Verification items for the finished model (mm, model axes). A direction names the side the tool comes from. Coordinates: 2 decimals unless noted, no trailing zeros. Write each loop counter-clockwise with the first axis right and the second up, starting at its lowest first coordinate (ties: lowest second). Pieces come first, ordered by that corner, then holes. Notation, with made-up numbers: (0.25, -19.5) -> (31.25, -19.5) arc R31 cw to (31.25, 11.5) -> close; hole circle Ø1 at (59.25, 83). An arc over 180 degrees is marked (long way). Write item = value, one per line. Start each with the question number.
(1) Section check A-A (x = 0). Record the cut outline in (y, z).
(2) Mould release check, pull along Z, two halves, no side actions. Record for faces 3 (the face through (0.29, -0.12, 76.25)), 4 (the face through (4, 0, 129.54)), 5 (the face through (0, 0, 0)): released by +Z, released by -Z, zero draft, split by the parting line, or undercut.
(3) Gauge pin test, flat ends, axial feed: pin 1 Ø2 at (x, z) = (0, 74.93) entering from -Y; pin 2 Ø8 at (x, z) = (-5.5, 101.5) entering from +Y; pin 3 Ø2 at (x, z) = (-5.5, 46.5) entering from -Y; pin 4 Ø1 at (x, y) = (5, -0.5) entering from +Z. Record the tip position at first contact, or that the pin passes through.
(4) Section check C-C (z = 125). Record the cut outline in (x, y).
(5) Section check B-B (y = 0). Record the cut outline in (x, z).
(6) Set-up check for faces 1 (the face through (0.29, -0.12, 109.27)), 2 (the face through (-2.3, -1.8, 138.3)): record each of +Z, -Z, +X, -X, +Y, -Y from which the full face is reachable in a straight line by a thin tool's end or side.
(7) Material ranges on probe 1 along Z at (x, y) = (0, 2); probe 2 along Z at (x, y) = (0, 0); probe 3 along Z at (x, y) = (0, 0.5), recorded low to high. Write a range as [from, to].
(8) Section check D-D (z = 107.95). Record the cut outline in (x, y), plus the area to 3 significant figures.
```python
from build123d import *

# Parameters (mm, degrees)
SKETCH1_R             = 8.73125
BOSS_EXTRUDE1_DEPTH   = 129.54
SKETCH2_R             = 2.921
BOSS_EXTRUDE2_DEPTH   = 17.78
F_6_32_TAPPED_HOLE1_D = 2.7051
F_6_32_TAPPED_HOLE2_D = 2.7051


with BuildPart() as part:
    # Sketch1 → Boss-Extrude1 (new body)
    with BuildSketch(Plane.XY):
        Circle(SKETCH1_R)
    extrude(amount=BOSS_EXTRUDE1_DEPTH)

    # Sketch2 → Boss-Extrude2 (add)
    with BuildSketch(Plane.XY.offset(129.54)):
        Circle(SKETCH2_R)
    extrude(amount=BOSS_EXTRUDE2_DEPTH)

    # #6-32 Tapped Hole1 (through all)
    with Locations(Plane(origin=(0, 8.73125, 0), x_dir=(1, 0, 0), z_dir=(0, 1, 0))):
        with Locations((0, -74.93), (0, -107.95)):
            Hole(F_6_32_TAPPED_HOLE1_D / 2)

    # #6-32 Tapped Hole2 (through all)
    with Locations(Plane(origin=(2.921, 0, 0), x_dir=(0, 0, -1), z_dir=(1, 0, 0))):
        with Locations((-138.43, 0)):
            Hole(F_6_32_TAPPED_HOLE2_D / 2)


solid = part.part
```
Response:
q1.outline = (-8.73, 0) -> (8.73, 0) -> (8.73, 73.58) -> (-8.73, 73.58) -> close; (-8.73, 76.28) -> (8.73, 76.28) -> (8.73, 106.6) -> (-8.73, 106.6) -> close; (-8.73, 109.3) -> (8.73, 109.3) -> (8.73, 129.54) -> (2.92, 129.54) -> (2.92, 147.32) -> (-2.92, 147.32) -> (-2.92, 129.54) -> (-8.73, 129.54) -> close; hole circle Ø2.71 at (0, 138.43)
q2.face_3 = undercut
q2.face_4 = released by +Z
q2.face_5 = released by -Z
q3.pin_1 = through
q3.pin_2 = 8.6
q3.pin_3 = -7.48
q3.pin_4 = 129.54
q4.outline = circle Ø17.46 at (0, 0)
q5.outline = (-8.73, 0) -> (8.73, 0) -> (8.73, 129.54) -> (2.92, 129.54) -> (2.92, 137.08) -> (-2.92, 137.08) -> (-2.92, 129.54) -> (-8.73, 129.54) -> close; (-2.92, 139.78) -> (2.92, 139.78) -> (2.92, 147.32) -> (-2.92, 147.32) -> close; hole circle Ø2.71 at (0, 74.93); hole circle Ø2.71 at (0, 107.95)
q6.face_1 = +Y, -Y
q6.face_2 = +Z
q7.probe_1 = [0, 73.58], [76.28, 106.6], [109.3, 147.32]
q7.probe_2 = [0, 73.58], [76.28, 106.6], [109.3, 137.08], [139.78, 147.32]
q7.probe_3 = [0, 73.58], [76.28, 106.6], [109.3, 137.17], [139.69, 147.32]
q8.outline = (-1.35, -8.63) -> (-1.35, 8.63) arc R8.73 ccw to start; (1.35, -8.63) arc R8.73 ccw to (1.35, 8.63) -> close
q8.area = 192 mm2
